Geometry check sheet. Reference: the model listing, model coordinates, mm. Coordinates: 2 decimals unless noted, no trailing zeros. Write each loop counter-clockwise with the first axis right and the second up, starting at its lowest first coordinate (ties: lowest second). Pieces come first, ordered by that corner, then holes. Notation, with made-up numbers: (35.25, 10) -> (75.25, 10) arc R22 ccw to (75.25, 44) -> close; hole circle Ø7 at (73, 59.5). An arc over 180 degrees is marked (long way). Use a Markdown table: item, result.
```python
from build123d import *

# Parameters (mm, degrees)
SKETCH1_R           = 6
SKETCH1_W           = 4
SKETCH1_H           = 25
BOSS_EXTRUDE1_DEPTH = 4


with BuildPart() as part:
    # Sketch1 → Boss-Extrude1 (new body)
    # profile 1 of 5: a face of its own
    with BuildSketch(Plane(origin=(0, 0, 0), x_dir=(1, 0, 0), z_dir=(0, 1, 0))):
        Polygon((0, 25), (0, 0), (200, 0), (200, 25), (200, 45), (200, 70), (0, 70), (0, 45), align=None)
        with Locations(Location((175, 10, 0), (0, 0, 270))):
            Circle(SKETCH1_R, mode=Mode.SUBTRACT)
    # profile 2 of 5: a face of its own
    with BuildSketch(Plane(origin=(0, 0, 0), x_dir=(1, 0, 0), z_dir=(0, 1, 0))):
        with Locations((-2, 12.5)):
            Rectangle(SKETCH1_W, SKETCH1_H)
    # profile 3 of 5: a face of its own
    with BuildSketch(Plane(origin=(0, 0, 0), x_dir=(1, 0, 0), z_dir=(0, 1, 0))):
        with Locations((202, 12.5)):
            Rectangle(SKETCH1_W, SKETCH1_H)
    # profile 4 of 5: a face of its own
    with BuildSketch(Plane(origin=(0, 0, 0), x_dir=(1, 0, 0), z_dir=(0, 1, 0))):
        with Locations((-2, 57.5)):
            Rectangle(SKETCH1_W, SKETCH1_H)
    # profile 5 of 5: a face of its own
    with BuildSketch(Plane(origin=(0, 0, 0), x_dir=(1, 0, 0), z_dir=(0, 1, 0))):
        with Locations((202, 57.5)):
            Rectangle(SKETCH1_W, SKETCH1_H)
    extrude(amount=BOSS_EXTRUDE1_DEPTH)


solid = part.part
```
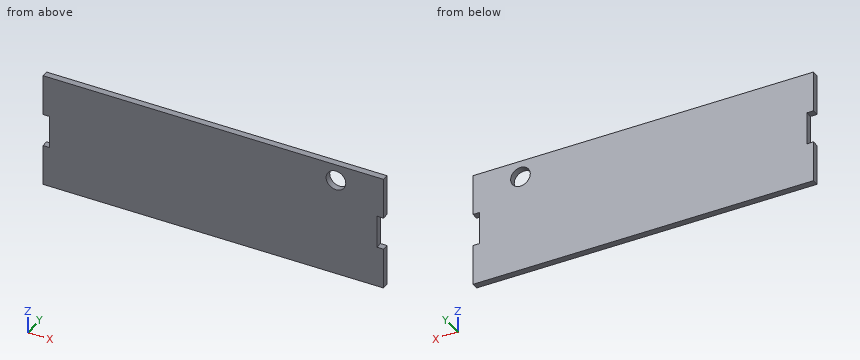
Item 1: Depth check by flat-ended pin: P1, Ø2, axis at x = -2.5, y = 1.5, coming from the +Z side; P2, Ø1.2, axis at y = 2, z = -39, coming from the -X side. Enter the tip coordinate at first touch or a pass-through.
Answer block:
| item | result |
|---|---|
| P1 | stops at z = 0 |
| P2 | stops at x = 0 |
Item 2: Section check C-C on y = 2.25. Record the boundary of the cut face in (x, z).
Answer block:
| item | result |
|---|---|
| outline | (-4, -70) -> (204, -70) -> (204, -45) -> (200, -45) -> (200, -25) -> (204, -25) -> (204, 0) -> (-4, 0) -> (-4, -25) -> (0, -25) -> (0, -45) -> (-4, -45) -> close; hole circle Ø12 at (175, -10) |
Item 3: Thickness scan on L1, parallel to X at y = 2, z = -10; L2, parallel to X at y = 1.4, z = -27.5; L3, parallel to X at y = 0.9, z = -9. Record the ranges inside material, lowest first. Write a range as [from, to].
Answer block:
| item | result |
|---|---|
| L1 | x = [-4, 169], [181, 204] |
| L2 | x = [0, 200] |
| L3 | x = [-4, 169.08], [180.92, 204] |
Item 4: Section check B-B on z = -10. Record the boundary of the cut face in (x, y).
Answer block:
| item | result |
|---|---|
| outline | (-4, 0) -> (169, 0) -> (169, 4) -> (-4, 4) -> close; (181, 0) -> (204, 0) -> (204, 4) -> (181, 4) -> close |
Item 5: Section check A-A on x = 175. Record the boundary of the cut face in (y, z).
Answer block:
| item | result |
|---|---|
| outline | (0, -70) -> (4, -70) -> (4, -16) -> (0, -16) -> close; (0, -4) -> (4, -4) -> (4, 0) -> (0, 0) -> close |
